Could you check a few things on this drawing? It's one solid part, dimensions in mm from its lowest x, y, z. A direction names the side the tool comes from. Round coordinates to 2 decimals unless told otherwise and drop trailing zeros. Loops run counter-clockwise (first coordinate to the right, second up) from the corner with the lowest first, then second, coordinate; pieces in that order, holes last. Notation, with made-up numbers: M -26,-28.5 L 32,-28.5 A24 cw 32,-2.5 Z; hole C 26.5,60.25 d5. An arc over 180 degrees is marked long. Answer as CSV lines item,"result".
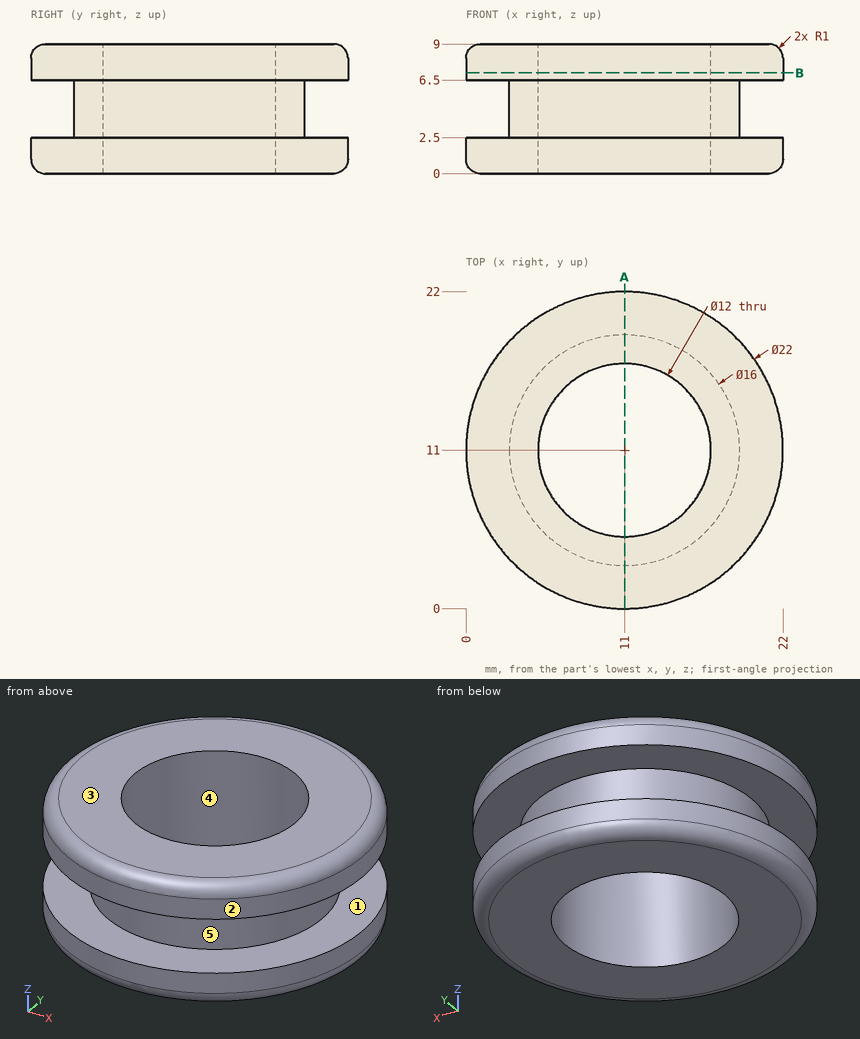
Item 1: If I drill on line 1 along Y through (x, z) = (11, 3); line 2 along Z through (x, y) = (21, 11.5); line 3 along Y through (x, z) = (11, 2), over which ranges is the centre line in solid material (lowest first)? Write a range as from..to.
Output:
line 1,"y = 3..5, 17..19"
line 2,"z = 0..2.5, 6.5..9"
line 3,"y = 0..5, 17..22"
Item 2: If we section it at A-A on x = 11: Write out the boundary of the cut face in (y, z), then the cut area to 3 significant figures.
Output:
outline,"M 0,1 A1 ccw 1,0 L 5,0 L 5,9 L 1,9 A1 ccw 0,8 L 0,6.5 L 3,6.5 L 3,2.5 L 0,2.5 Z; M 17,0 L 21,0 A1 ccw 22,1 L 22,2.5 L 19,2.5 L 19,6.5 L 22,6.5 L 22,8 A1 ccw 21,9 L 17,9 Z"
area,"65.1 mm2"
Item 3: Will this pin go through, and if not, where does the flat tip stop? pin 1 (5 mm diameter, centred on x = 15.5, z = 8, fed in from -Y).
Output:
pin 1,"stops at y = 0.18"
Item 4: We'd pull the mould along Z, two halves only. Please class the marked faces 3, 4 and 5: released by +Z, released by -Z, zero draft, split by the parting line, or undercut.
Output:
face 3,"released by +Z"
face 4,"zero draft"
face 5,"undercut"
Item 5: If we section it at B-B on z = 7: Write out the boundary of the cut face in (x, y).
Output:
outline,"C 11,11 d22; hole C 11,11 d12"
Item 6: On a 3-axis mill with a long thin cutter (end or side, diameter ignored), from which of +Z, -Z, +X, -X, +Y, -Y can I reach the whole of each face in a straight line? I mean the marked faces 1 and 2. Say none if no direction works.
Output:
face 1,"none"
face 2,"+Z, -Z"
